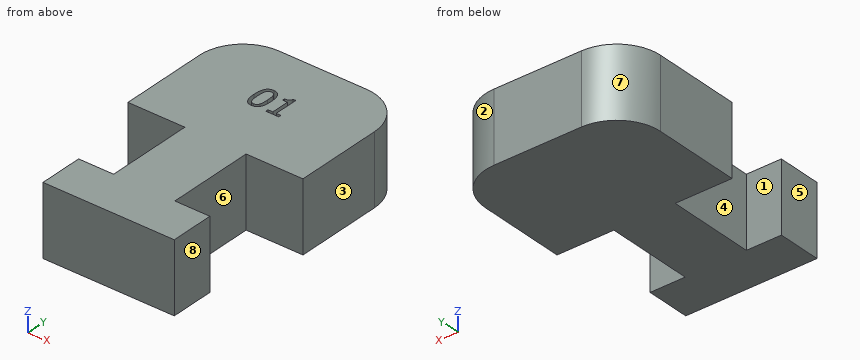
Autodesk Inventor part; units mm, degrees
ref_plane "YZ Plane" through (0, 0, 0) normal (1, 0, 0) x (0, 1, 0)
ref_plane "XZ Plane" through (0, 0, 0) normal (0, 1, 0) x (-1, 0, 0)
ref_plane "XY Plane" through (0, 0, 0) normal (0, 0, 1) x (1, 0, 0)
sketch "스케치1" plane through (0, 0, 0) normal (0, 0, 1) x (1, 0, 0)
  line L0 (-5, 14) -> (5, 14)
  line L1 (7.5, -16.0251) -> (-7.5, -16.0251)
  line L2 (-7.5, -11.0251) -> (-7.5, -16.0251)
  line L3 (3.5, -1.0251) -> (3.5, -11.0251)
  line L4 (-3.5, -11.0251) -> (-3.5, -1.0251)
  line L5 (7.5, -11.0251) -> (7.5, -16.0251)
  line L6 (-3.5, -1.0251) -> (-10, -1.0251)
  line L7 (-3.5, -1.0251) -> (3, -1.0251) construction
  line L8 (3.5, -1.0251) -> (10, -1.0251)
  line L9 (3.5, -1.0251) -> (10, -1.0251) construction
  line L10 (-10, 9) -> (-10, -1.0251)
  line L11 (10, -1.0251) -> (10, 9)
  line L12 (-7.5, -11.0251) -> (-3.5, -11.0251)
  line L13 (3.5, -11.0251) -> (7.5, -11.0251)
  arc A0 (-5, 14) -> (-10, 9) centre (-5, 9) ccw
  arc A1 (10, 9) -> (5, 14) centre (5, 9) ccw
  point P0 (0, 0)
  point P1 (-10, 14)
  point P2 (10, 14)
  dimension "d2" = 20
  dimension "d5" = 15
  dimension "d7" = 7.5
  dimension "d12" = 7
  dimension "d13" = 3.5
  dimension "d14" = 180
  dimension "d15" = 0
  dimension "d16" = 5
  dimension "d17" = 5
  dimension "d18" = 10
sketch "스케치2" plane through (0, 0, 0) normal (0, 0, 1) x (1, 0, 0)
  line L0 (10, -1) -> (3.4836, -1)
  point P0 (0, 0)
sketch "스케치3" plane through (0, 0, 0) normal (0, 0, 1) x (1, 0, 0)
  point P0 (0, 0)
extrude "돌출1" add sketch "스케치1" along normal blind 8
sketch "스케치4" plane through (0, 0, 8) normal (0, 0, 1) x (1, 0, 0)
  line L0 (-2.3546, 8.6646) -> (2.2199, 8.6646) construction
  line L1 (2.2199, 8.6646) -> (2.2199, 5.4907) construction
  line L2 (2.2199, 5.4907) -> (-2.3546, 5.4907) construction
  line L3 (-2.3546, 5.4907) -> (-2.3546, 8.6646) construction
  spline S0 degree 2 poles (-0.2353, 7.0789) (-0.2353, 6.2588) (-0.712, 5.4907) (-1.2085, 5.4907) knots 0 0 0 1 2 2 2
  spline S1 degree 2 poles (-1.2085, 5.4907) (-1.7124, 5.4907) (-2.1841, 6.2737) (-2.1841, 7.0764) knots 0 0 0 1 2 2 2
  spline S2 degree 2 poles (-2.1841, 7.0764) (-2.1841, 7.9014) (-1.7074, 8.6646) (-1.2085, 8.6646) knots 0 0 0 1 2 2 2
  spline S3 degree 2 poles (-1.2085, 8.6646) (-0.7071, 8.6646) (-0.2353, 7.8742) (-0.2353, 7.0789) knots 0 0 0 1 2 2 2
  spline S4 degree 2 poles (-0.7589, 6.1502) (-0.6997, 6.3008) (-0.6503, 6.7652) (-0.6503, 7.0789) knots 0 0 0 1 2 2 2
  spline S5 degree 2 poles (-0.6503, 7.0789) (-0.6503, 7.3926) (-0.6997, 7.8545) (-0.7614, 8.0101) knots 0 0 0 1 2 2 2
  spline S6 degree 2 poles (-0.7614, 8.0101) (-0.8232, 8.1657) (-1.0381, 8.3263) (-1.2085, 8.3263) knots 0 0 0 1 2 2 2
  spline S7 degree 2 poles (-1.2085, 8.3263) (-1.3789, 8.3263) (-1.5988, 8.1657) (-1.663, 8.0052) knots 0 0 0 1 2 2 2
  spline S8 degree 2 poles (-1.663, 8.0052) (-1.7247, 7.8495) (-1.7692, 7.3753) (-1.7692, 7.0764) knots 0 0 0 1 2 2 2
  spline S9 degree 2 poles (-1.7692, 7.0764) (-1.7692, 6.7553) (-1.7297, 6.3255) (-1.6654, 6.1576) knots 0 0 0 1 2 2 2
  spline S10 degree 2 poles (-1.6654, 6.1576) (-1.6062, 5.9995) (-1.3863, 5.8291) (-1.2085, 5.8291) knots 0 0 0 1 2 2 2
  spline S11 degree 2 poles (-1.2085, 5.8291) (-1.0405, 5.8291) (-0.8207, 5.9896) (-0.7589, 6.1502) knots 0 0 0 1 2 2 2
  line L4 (1.8815, 5.5549) -> (0.3945, 5.5549)
  line L5 (0.3945, 5.5549) -> (0.3945, 5.8661)
  line L6 (0.3945, 5.8661) -> (0.9478, 5.8661)
  line L7 (0.9478, 5.8661) -> (0.9478, 7.9088)
  line L8 (0.9478, 7.9088) -> (0.3945, 7.9088)
  line L9 (0.3945, 7.9088) -> (0.3945, 8.1879)
  spline S12 degree 2 poles (0.3945, 8.1879) (0.7082, 8.1879) (1.0046, 8.3658) (1.0244, 8.6128) knots 0 0 0 1 2 2 2
  line L10 (1.0244, 8.6128) -> (1.3406, 8.6128)
  line L11 (1.3406, 8.6128) -> (1.3406, 5.8661)
  line L12 (1.3406, 5.8661) -> (1.8815, 5.8661)
  line L13 (1.8815, 5.8661) -> (1.8815, 5.5549)
  point P0 (0, 0)
extrude "돌출2" cut sketch "스케치4" against normal blind 3
properties part number "01_02"
Source: CAD feature listing. Evaluate the final solid. Frame: model axes, mm. Face numbers are marked on the shaded views. A direction names the side the tool comes from. Give positions to 0.01 mm unless a question says otherwise; leave off trailing zeros. Loops run counter-clockwise (first coordinate to the right, second up) from the corner with the lowest first, then second, coordinate; pieces in that order, holes last. Notation, with made-up numbers: (50.5, 89.25) - (108.5, 89.25) arc R29 cw to (108.5, 124.25) - close; hole circle Ø2 at (89.5, 81). An arc over 180 degrees is marked (long way). Use CSV: the item, a comma, the result in double quotes.
1) Set-up query: the marked faces 4, 5, 6, 7 and 8. Return all of +Z, -Z, +X, -X, +Y, -Y with unobstructed straight access to the full face (end or side cutting, diameter ignored); none if empty.
Worked out:
face 4,"+Z, -Z, -X"
face 5,"+Z, -Z, -X, -Y"
face 6,"+Z, -Z, +X"
face 7,"+Z, -Z, -X, +Y"
face 8,"+Z, -Z, +X, -Y"
2) Cut plane C-C (y = -12.5). Output: boundary loops of the cut face in (x, z).
Worked out:
outline,"(-7.5, 0) - (7.5, 0) - (7.5, 8) - (-7.5, 8) - close"
3) Cut plane D-D (z = 4.5). Output: boundary loops of the cut face in (x, y).
Worked out:
outline,"(-10, -1.03) - (-3.5, -1.03) - (-3.5, -11.03) - (-7.5, -11.03) - (-7.5, -16.03) - (7.5, -16.03) - (7.5, -11.03) - (3.5, -11.03) - (3.5, -1.03) - (10, -1.03) - (10, 9) arc R5 ccw to (5, 14) - (-5, 14) arc R5 ccw to (-10, 9) - close"
4) Pin query (flat end, axial travel): P1, Ø4, axis at y = -12, z = 1.5, coming from the -X side. Return the tip coordinate at first contact, or that it passes through.
Worked out:
P1,"stops at x = -7.5"
5) Line query: line 1 (Y direction, x = -3.75, z = 7); line 2 (X direction, y = -15, z = 7.25); line 3 (X direction, y = -9.5, z = 4.5). Output: solid intervals per line, ascending.
Worked out:
line 1,"y = -16.03 to -11.03, -1.03 to 14"
line 2,"x = -7.5 to 7.5"
line 3,"x = -3.5 to 3.5"
6) Cut plane A-A (x = 5.75). Output: boundary loops of the cut face in (y, z), and give its area (3 significant figures).
Worked out:
outline,"(-16.03, 0) - (-11.03, 0) - (-11.03, 8) - (-16.03, 8) - close; (-1.03, 0) - (13.94, 0) - (13.94, 8) - (-1.03, 8) - close"
area,"160 mm^2"
7) Mould query, pull axis Y, two halves, no side actions, for the marked faces 1, 2 and 3. Classes: +Y half, -Y half, draft (parallel to the pull), parting line (faces both ways), or undercut.
Worked out:
face 1,"undercut"
face 2,"+Y half"
face 3,"draft"
8) Cut plane B-B (z = 6). Count the separate pieces of the cut face and the enclosed holes in it, and give its area (3 significant figures).
Worked out:
separate pieces,"2"
enclosed holes,"2"
area,"430 mm^2"
